Build history of the part. All positions in model axes, mm. Face numbers are marked on the shaded views. A direction names the side the tool comes from. Round coordinates to 2 decimals unless told otherwise and drop trailing zeros. Write each loop counter-clockwise with the first axis right and the second up, starting at its lowest first coordinate (ties: lowest second). Pieces come first, ordered by that corner, then holes. Notation, with made-up numbers: M 87,-28.75 L 120,-28.75 A26 ccw 120,1.25 Z; hole C 27.5,-35.5 d8. An arc over 180 degrees is marked long. Write item = value, one per line. Start each with the question number.
Q1. Tool access for the marked faces 1, 2 and 3: list every direction of +Z, -Z, +X, -X, +Y, -Y with a clear straight run to the whole face (end or side of a thin tool).
Q2. Band-saw the part on D-D on y = -1. Write the cut outline in (x, z), plus the area to 3 significant figures.
Q3. Band-saw the part on B-B on y = -23.5. Write the cut outline in (x, z), plus the area to 3 significant figures.
Q4. Probe L1, parallel to Y at x = 37, z = 8; L2, parallel to Y at x = -2.5, z = 9.5; L3, parallel to Z at x = 29.5, y = 16. List the from-to ranges inside material, lowest first.
Q5. Pull direction Y, two halves, no side cores. Call the marked faces 4, 5 and 6: released by +Y, released by -Y, zero draft, split by the parting line, or undercut.
Q6. Band-saw the part on C-C on z = 4. Write the cut outline in (x, y), plus the area to 3 significant figures.
Q7. Band-saw the part on A-A on x = -1. Write the cut outline in (y, z).
Q8. Drop flat-ended pins along their axis: P1, Ø11.5, axis at x = -3.96, y = -26.39, coming from the +Z side; P2, Ø1.5, axis at y = 12, z = 13.5, coming from the -X side; P3, Ø7, axis at x = 41.5, z = 21.5, coming from the -Y side. Give the stop position or say it passes through.
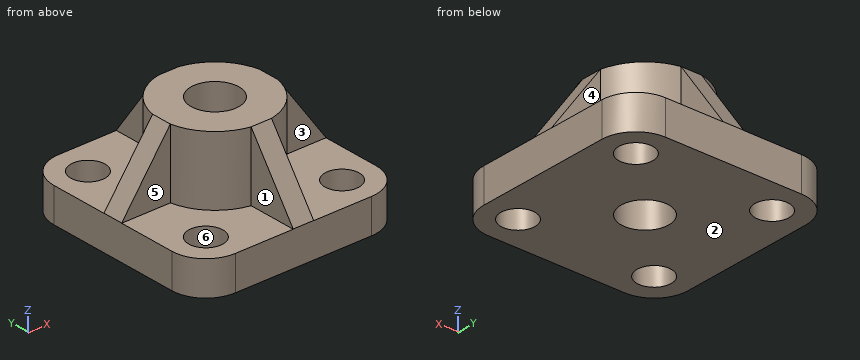
```python
from build123d import *

# Parameters (mm, degrees)
F0_W     = 60
F0_H     = 60
F1_DEPTH = 10
F2_R     = 10
F4_D     = 10
F5_DEPTH = 20
F7_D     = 14
F7_DEPTH = 31
F7_TIP   = 4.2060243332
F8_SIZE2 = 19.9516800852
F8_SIZE  = 14.284


with BuildPart() as f1:
    # F0 (on Top) → F1 (new body)
    with BuildSketch(Plane.XY):
        with Locations((16.0370518267, -6.3885685802)):
            Rectangle(F0_W, F0_H)
    extrude(amount=F1_DEPTH)

    # F2
    f2_edges = [f1.edges().sort_by_distance(p)[0] for p in [
        (-13.962948, 23.611431, 5),
        (46.037052, 23.611431, 5),
        (46.037052, -36.388569, 5),
        (-13.962948, -36.388569, 5),
    ]]
    fillet(f2_edges, radius=F2_R)

    # F4 (through all)
    with Locations(Plane.XY.offset(10)):
        with Locations((-3.9629481733, 13.6114314198), (36.0370518267, 13.6114314198), (36.0370518267, -26.3885685802), (-3.9629481733, -26.3885685802)):
            Hole(F4_D / 2)

    # F3 (on face) → F5 (join)
    with BuildSketch(Plane.XY.offset(10)):
        with BuildLine():
            ThreePointArc((31.7535637154, -9.3888022257), (31.9662305079, -7.8954975618), (32.0373300699, -6.3888022257))
            ThreePointArc((32.0373300699, -6.3888022257), (31.9662305079, -4.8821068895), (31.7535637154, -3.3888022257))
            ThreePointArc((31.7535637154, -3.3888022257), (27.3510385689, 4.9249062733), (19.0373300699, 9.3274314198))
            ThreePointArc((19.0373300699, 9.3274314198), (16.0373300699, 9.6111977743), (13.0373300699, 9.3274314198))
            ThreePointArc((13.0373300699, 9.3274314198), (4.723621571, 4.9249062733), (0.3210964244, -3.3888022257))
            ThreePointArc((0.3210964244, -3.3888022257), (0.0373300704, -6.3886832938), (0.3210518267, -9.3885685802))
            ThreePointArc((0.3210518267, -9.3885685802), (4.7235374737, -17.7024266268), (13.0373300699, -22.1050358712))
            ThreePointArc((13.0373300699, -22.1050358712), (16.0373300699, -22.3888022257), (19.0373300699, -22.1050358712))
            ThreePointArc((19.0373300699, -22.1050358712), (27.3510385689, -17.7025107246), (31.7535637154, -9.3888022257))
        make_face()
        with BuildLine():
            ThreePointArc((31.7535637154, -3.3888022257), (31.9662305079, -4.8821068895), (32.0373300699, -6.3888022257))
            ThreePointArc((32.0373300699, -6.3888022257), (31.9662305079, -7.8954975618), (31.7535637154, -9.3888022257))
            Line((31.7535637154, -9.3888022257), (46.0370518267, -9.3888022257))
            Line((46.0370518267, -9.3888022257), (46.0370518267, -6.3885685802))
            Line((46.0370518267, -6.3885685802), (46.0370518267, -3.3888022257))
            Line((46.0370518267, -3.3888022257), (31.7535637154, -3.3888022257))
        make_face()
        with BuildLine():
            ThreePointArc((13.0373300699, 9.3274314198), (16.0373300699, 9.6111977743), (19.0373300699, 9.3274314198))
            Line((19.0373300699, 9.3274314198), (19.0373300699, 23.6114314198))
            Line((19.0373300699, 23.6114314198), (16.0370518267, 23.6114314198))
            Line((16.0370518267, 23.6114314198), (13.0373300699, 23.6114314198))
            Line((13.0373300699, 23.6114314198), (13.0373300699, 9.3274314198))
        make_face()
        with BuildLine():
            Line((19.0373300699, -36.3885685802), (19.0373300699, -22.1050358712))
            ThreePointArc((19.0373300699, -22.1050358712), (16.0373300699, -22.3888022257), (13.0373300699, -22.1050358712))
            Line((13.0373300699, -22.1050358712), (13.0373300699, -36.3885685802))
            Line((13.0373300699, -36.3885685802), (16.0370518267, -36.3885685802))
            Line((16.0370518267, -36.3885685802), (19.0373300699, -36.3885685802))
        make_face()
        with BuildLine():
            ThreePointArc((0.3210518267, -9.3885685802), (0.0373300704, -6.3886832938), (0.3210964244, -3.3888022257))
            Line((0.3210964244, -3.3888022257), (-13.9629481733, -3.3888022257))
            Line((-13.9629481733, -3.3888022257), (-13.9629481733, -6.3885685802))
            Line((-13.9629481733, -6.3885685802), (-13.9629481733, -9.3885685802))
            Line((-13.9629481733, -9.3885685802), (0.3210518267, -9.3885685802))
        make_face()
    extrude(amount=F5_DEPTH)

    # F7
    with Locations(Plane.XY.offset(30)):
        with Locations((16.0373300699, -6.3888022257)):
            Hole(F7_D / 2, depth=F7_DEPTH)
            with Locations((0, 0, -(F7_DEPTH + F7_TIP / 2))):  # 118° drill point
                Cone(0, F7_D / 2, F7_TIP, mode=Mode.SUBTRACT)

    # F8
    f8_edges = [f1.edges().sort_by_distance(p)[0] for p in [
        (-13.962948, -6.388685, 30),
        (16.03733, 23.611431, 30),
        (46.037052, -6.388802, 30),
        (16.03733, -36.388569, 30),
    ]]
    f8_side = f1.faces().sort_by_distance((26.751039, 4.324906, 30))[0]
    chamfer(f8_edges, length=F8_SIZE, length2=F8_SIZE2, reference=f8_side)


solid = f1.part
```
Conclusion:
q1.face_1 = +Z, -X, -Y
q1.face_2 = -Z, +X, -X, +Y, -Y
q1.face_3 = +Z, +X, -Y
q2.outline = M -13.96,0 L 11.57,0 L 11.57,30 L 0.97,30 L 0.97,10 L -13.96,10 Z; M 20.51,0 L 46.04,0 L 46.04,10 L 31.1,10 L 31.1,30 L 20.51,30 Z
q2.area = 935 mm^2
q3.outline = M -13.96,0 L -8.04,0 L -8.04,10 L -13.96,10 Z; M 0.12,0 L 31.96,0 L 31.96,10 L 19.04,10 L 19.04,28.05 L 13.04,28.05 L 13.04,10 L 0.12,10 Z; M 40.12,0 L 46.04,0 L 46.04,10 L 40.12,10 Z
q3.area = 545 mm^2
q4.L1 = -36.34 to -31.29, -21.48 to 8.71, 18.52 to 23.56
q4.L2 = -36.39 to -31.17, -21.61 to 8.83, 18.39 to 23.61
q4.L3 = 0 to 10
q5.face_4 = released by +Y
q5.face_5 = released by -Y
q5.face_6 = undercut
q6.outline = M -13.96,-26.39 A10 ccw -3.96,-36.39 L 36.04,-36.39 A10 ccw 46.04,-26.39 L 46.04,13.61 A10 ccw 36.04,23.61 L -3.96,23.61 A10 ccw -13.96,13.61 Z; hole C -3.96,-26.39 d10; hole C -3.96,13.61 d10; hole C 16.04,-6.39 d14; hole C 36.04,-26.39 d10; hole C 36.04,13.61 d10
q6.area = 3,050 mm^2
q7.outline = M -36.39,0 L -30.42,0 L -30.42,10 L -36.39,10 Z; M -22.36,0 L 9.58,0 L 9.58,10 L -3.39,10 L -3.39,28.15 L -9.39,28.15 L -9.39,10 L -22.36,10 Z; M 17.64,0 L 23.61,0 L 23.61,10 L 17.64,10 Z
q8.P1 = 10
q8.P2 = 13.04
q8.P3 = -9.39
